Check sheet for the modelled part. Datum: model origin and axes. Units: mm. Face numbers are marked on the shaded views. A direction names the side the tool comes from. Coordinates: 2 decimals unless noted, no trailing zeros. Loops run counter-clockwise (first coordinate to the right, second up) from the corner with the lowest first, then second, coordinate; pieces in that order, holes last. Notation, with made-up numbers: (40, -22.75) -> (70, -22.75) arc R14 cw to (70, -8.75) -> close; hole circle Ø11 at (16, -8). An arc over 180 degrees is marked (long way). Use CSV: the item, a comma, the result in double quotes.
```python
from build123d import *

# Parameters (mm, degrees)
ESQUISSE1_R        = 11
BOSS_EXTRU_1_DEPTH = 5
BOSS_EXTRU_3_DEPTH = 5
CONG_3_R           = 0.5


with BuildPart() as part:
    # Esquisse1 → Boss.-Extru.1 (new body)
    with BuildSketch(Plane.XY):
        Circle(ESQUISSE1_R)
    extrude(amount=BOSS_EXTRU_1_DEPTH)

    # Esquisse2 → Boss.-Extru.3 (add)
    with BuildSketch(Plane.XY.offset(5)):
        with BuildLine():
            ThreePointArc((-2.5, 10.712142643), (-5.174562286, 9.706899873), (-7.5, 8.04673847))
            Line((-7.5, 8.04673847), (-7.5, -8.04673847))
            ThreePointArc((-7.5, -8.04673847), (-5.174562286, -9.706899873), (-2.5, -10.712142643))
            Line((-2.5, -10.712142643), (-2.5, 10.712142643))
        make_face()
        with BuildLine():
            ThreePointArc((7.5, 8.04673847), (5.174562286, 9.706899873), (2.5, 10.712142643))
            Line((2.5, 10.712142643), (2.5, -10.712142643))
            ThreePointArc((2.5, -10.712142643), (5.174562286, -9.706899873), (7.5, -8.04673847))
            Line((7.5, -8.04673847), (7.5, 8.04673847))
        make_face()
    extrude(amount=BOSS_EXTRU_3_DEPTH)

    # Congé3
    cong_3_edges = [part.edges().sort_by_distance(p)[0] for p in [
        (5.174562286, 9.706899873, 10),
        (5.174562286, -9.706899873, 10),
        (7.5, 0, 10),
        (2.5, 0, 10),
        (-5.174562286, 9.706899873, 10),
        (-5.174562286, -9.706899873, 10),
        (-2.5, 0, 10),
        (-7.5, 0, 10),
    ]]
    fillet(cong_3_edges, radius=CONG_3_R)


solid = part.part
```
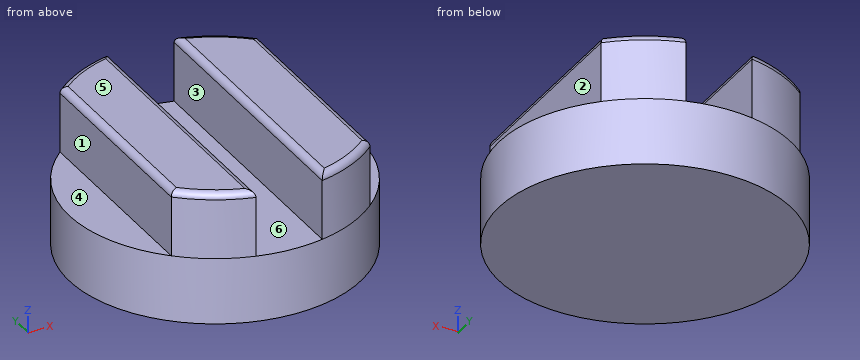
1) Cross-section at C-C on x = 0. Record the boundary of the cut face in (y, z), and give its area (3 significant figures).
Answer below:
outline,"(-11, 0) -> (11, 0) -> (11, 5) -> (-11, 5) -> close"
area,"110 mm²"
2) Cross-section at A-A on z = 6.75. Record the boundary of the cut face in (x, y).
Answer below:
outline,"(-7.5, -8.05) arc R11 ccw to (-2.5, -10.71) -> (-2.5, 10.71) arc R11 ccw to (-7.5, 8.05) -> close; (2.5, -10.71) arc R11 ccw to (7.5, -8.05) -> (7.5, 8.05) arc R11 ccw to (2.5, 10.71) -> close"
3) Access from +Z, -Z, +X, -X, +Y, -Y to the whole of each face (thin tool, end or side, straight path). Record for the marked faces 5 and 6.
Answer below:
face 5,"+Z, +X, -X, +Y, -Y"
face 6,"+Z, +Y, -Y"
4) Cross-section at D-D on z = 4.5. Record the boundary of the cut face in (x, y), and give its area (3 significant figures).
Answer below:
outline,"circle Ø22 at (0, 0)"
area,"380 mm²"
5) Thickness scan on line 1 along X through (y, z) = (6.25, 6.25); line 2 along Z through (x, y) = (-2, -8.25); line 3 along Y through (x, z) = (-2.5, 2.5). Record the ranges inside material, lowest first. Write a range as from..to.
Answer below:
line 1,"x = -7.5..-2.5, 2.5..7.5"
line 2,"z = 0..5"
line 3,"y = -10.71..10.71"
6) Go/stop test with flat-tipped pins: pin 1 Ø2 at (y, z) = (-3.5, 7.5) entering from -X; pin 2 Ø5 at (x, z) = (-6.5, 6) entering from +Y; pin 3 Ø5 at (x, z) = (6, 4.5) entering from -Y. Record where each tip stops, or that it passes through.
Answer below:
pin 1,"stops at x = -7.5"
pin 2,"stops at y = 10.25"
pin 3,"stops at y = -10.43"
7) Cross-section at B-B on y = 0. Record the boundary of the cut face in (x, z), and give its area (3 significant figures).
Answer below:
outline,"(-11, 0) -> (11, 0) -> (11, 5) -> (7.5, 5) -> (7.5, 9.5) arc R0.5 ccw to (7, 10) -> (3, 10) arc R0.5 ccw to (2.5, 9.5) -> (2.5, 5) -> (-2.5, 5) -> (-2.5, 9.5) arc R0.5 ccw to (-3, 10) -> (-7, 10) arc R0.5 ccw to (-7.5, 9.5) -> (-7.5, 5) -> (-11, 5) -> close"
area,"160 mm²"
8) Draft check along X on the marked faces 1, 2, 3 and 4. Enter one of: released by +X, released by -X, zero draft, split by the parting line, or undercut.
Answer below:
face 1,"released by -X"
face 2,"released by +X"
face 3,"undercut"
face 4,"zero draft"
